```python
from build123d import *

# Parameters (mm, degrees)
SKETCH1_R           = 2
SKETCH1_R_2         = 15
BOSS_EXTRUDE1_DEPTH = 5
FILLET1_R           = 3


with BuildPart() as part:
    # Sketch1 → Boss-Extrude1 (new body)
    with BuildSketch(Plane.XY):
        Polygon((-19.5, -21), (19.5, -21), (19.5, -54), (29.5, -54), (29.5, -17.031832941), (61.515371804, 1.452250588), (56.515371804, 10.112504626), (27.936533479, -6.387495374), (8.436533479, 27.387495374), (37.015371804, 43.887495374), (32.015371804, 52.547749412), (0, 34.063665882), (-32.015371804, 52.547749412), (-37.015371804, 43.887495374), (-8.436533479, 27.387495374), (-27.936533479, -6.387495374), (-56.515371804, 10.112504626), (-61.515371804, 1.452250588), (-29.5, -17.031832941), (-29.5, -54), (-19.5, -54), align=None)
        with Locations((24.5, -24)):
            Circle(SKETCH1_R, mode=Mode.SUBTRACT)
        with Locations((24.5, -29)):
            Circle(SKETCH1_R, mode=Mode.SUBTRACT)
        with Locations((24.5, -34)):
            Circle(SKETCH1_R, mode=Mode.SUBTRACT)
        with Locations((24.5, -39)):
            Circle(SKETCH1_R, mode=Mode.SUBTRACT)
        with Locations((24.5, -44)):
            Circle(SKETCH1_R, mode=Mode.SUBTRACT)
        with Locations((24.5, -49)):
            Circle(SKETCH1_R, mode=Mode.SUBTRACT)
        with Locations(Location((-24.5, -49, 0), (0, 0, 180))):
            Circle(SKETCH1_R, mode=Mode.SUBTRACT)
        with Locations(Location((-24.5, -44, 0), (0, 0, 180))):
            Circle(SKETCH1_R, mode=Mode.SUBTRACT)
        with Locations(Location((-24.5, -39, 0), (0, 0, 180))):
            Circle(SKETCH1_R, mode=Mode.SUBTRACT)
        with Locations(Location((-24.5, -34, 0), (0, 0, 180))):
            Circle(SKETCH1_R, mode=Mode.SUBTRACT)
        with Locations(Location((-24.5, -29, 0), (0, 0, 180))):
            Circle(SKETCH1_R, mode=Mode.SUBTRACT)
        with Locations(Location((-24.5, -24, 0), (0, 0, 180))):
            Circle(SKETCH1_R, mode=Mode.SUBTRACT)
        with Locations(Location((-8.534609691, 33.217622393, 0), (0, 0, 180))):
            Circle(SKETCH1_R, mode=Mode.SUBTRACT)
        with Locations(Location((-12.86473671, 35.717622393, 0), (0, 0, 180))):
            Circle(SKETCH1_R, mode=Mode.SUBTRACT)
        with Locations(Location((-17.194863729, 38.217622393, 0), (0, 0, 180))):
            Circle(SKETCH1_R, mode=Mode.SUBTRACT)
        with Locations(Location((-21.524990748, 40.717622393, 0), (0, 0, 180))):
            Circle(SKETCH1_R, mode=Mode.SUBTRACT)
        with Locations(Location((-25.855117767, 43.217622393, 0), (0, 0, 180))):
            Circle(SKETCH1_R, mode=Mode.SUBTRACT)
        with Locations(Location((-30.185244785, 45.717622393, 0), (0, 0, 180))):
            Circle(SKETCH1_R, mode=Mode.SUBTRACT)
        with Locations((-33.034609691, -9.217622393)):
            Circle(SKETCH1_R, mode=Mode.SUBTRACT)
        with Locations((-37.36473671, -6.717622393)):
            Circle(SKETCH1_R, mode=Mode.SUBTRACT)
        with Locations((-41.694863729, -4.217622393)):
            Circle(SKETCH1_R, mode=Mode.SUBTRACT)
        with Locations((-46.024990748, -1.717622393)):
            Circle(SKETCH1_R, mode=Mode.SUBTRACT)
        with Locations((-50.355117767, 0.782377607)):
            Circle(SKETCH1_R, mode=Mode.SUBTRACT)
        with Locations((-54.685244785, 3.282377607)):
            Circle(SKETCH1_R, mode=Mode.SUBTRACT)
        with Locations(Location((33.034609691, -9.217622393, 0), (0, 0, 180))):
            Circle(SKETCH1_R, mode=Mode.SUBTRACT)
        with Locations(Location((37.36473671, -6.717622393, 0), (0, 0, 180))):
            Circle(SKETCH1_R, mode=Mode.SUBTRACT)
        with Locations(Location((41.694863729, -4.217622393, 0), (0, 0, 180))):
            Circle(SKETCH1_R, mode=Mode.SUBTRACT)
        with Locations(Location((46.024990748, -1.717622393, 0), (0, 0, 180))):
            Circle(SKETCH1_R, mode=Mode.SUBTRACT)
        with Locations(Location((50.355117767, 0.782377607, 0), (0, 0, 180))):
            Circle(SKETCH1_R, mode=Mode.SUBTRACT)
        with Locations(Location((54.685244785, 3.282377607, 0), (0, 0, 180))):
            Circle(SKETCH1_R, mode=Mode.SUBTRACT)
        with Locations((8.534609691, 33.217622393)):
            Circle(SKETCH1_R, mode=Mode.SUBTRACT)
        with Locations((12.86473671, 35.717622393)):
            Circle(SKETCH1_R, mode=Mode.SUBTRACT)
        with Locations((17.194863729, 38.217622393)):
            Circle(SKETCH1_R, mode=Mode.SUBTRACT)
        with Locations((21.524990748, 40.717622393)):
            Circle(SKETCH1_R, mode=Mode.SUBTRACT)
        with Locations((25.855117767, 43.217622393)):
            Circle(SKETCH1_R, mode=Mode.SUBTRACT)
        with Locations((30.185244785, 45.717622393)):
            Circle(SKETCH1_R, mode=Mode.SUBTRACT)
        with Locations((0, 20)):
            Circle(SKETCH1_R, mode=Mode.SUBTRACT)
        with Locations((17.320508076, -10)):
            Circle(SKETCH1_R, mode=Mode.SUBTRACT)
        with Locations((-17.320508076, -10)):
            Circle(SKETCH1_R, mode=Mode.SUBTRACT)
        Circle(SKETCH1_R_2, mode=Mode.SUBTRACT)
    extrude(amount=BOSS_EXTRUDE1_DEPTH)

    # Fillet1
    fillet1_edges = [part.edges().sort_by_distance(p)[0] for p in [
        (19.5, -54, 2.5),
        (19.5, -21, 2.5),
        (-19.5, -21, 2.5),
        (-19.5, -54, 2.5),
        (-29.5, -54, 2.5),
        (-29.5, -17.031832941, 2.5),
        (-61.515371804, 1.452250588, 2.5),
        (-56.515371804, 10.112504626, 2.5),
        (-27.936533479, -6.387495374, 2.5),
        (-8.436533479, 27.387495374, 2.5),
        (-37.015371804, 43.887495374, 2.5),
        (-32.015371804, 52.547749412, 2.5),
        (0, 34.063665882, 2.5),
        (32.015371804, 52.547749412, 2.5),
        (37.015371804, 43.887495374, 2.5),
        (8.436533479, 27.387495374, 2.5),
        (27.936533479, -6.387495374, 2.5),
        (56.515371804, 10.112504626, 2.5),
        (61.515371804, 1.452250588, 2.5),
        (29.5, -17.031832941, 2.5),
        (29.5, -54, 2.5),
    ]]
    fillet(fillet1_edges, radius=FILLET1_R)


solid = part.part
```
Design review of the part built by this model. Coordinates are the model's own, in mm. A direction names the side the tool comes from. Round coordinates to 2 decimals unless told otherwise and drop trailing zeros. Write each loop counter-clockwise with the first axis right and the second up, starting at its lowest first coordinate (ties: lowest second). Pieces come first, ordered by that corner, then holes.
Item 1: The part is to be moulded in two halves that separate along X. For faces 4 (the flat face through (22.56, 35.54, 2.46)), 5 (the cylindrical face through (-15.721, 36.866, 2.465)), say which applies: +X half, -X half, draft (parallel to the pull), parting line (faces both ways), or undercut.
Item 2: Clearance check with a flat-ended pin moving along its axis: pin 1 Ø2 at (y, z) = (-25, 2.5) entering from +X. State where the tip first meets the part, or that it passes through.
Item 3: We need section C-C on y = 20. Write out the cut boundary in (x, z), and give its area (3 significant figures).
Item 4: We need section A-A on x = 0. Write out the cut boundary in (y, z).
Item 5: We need section B-B on y = -29. Write out the cut boundary in (x, z).
Item 6: For probe 1 along Y at (x, z) = (-21, 2.2); probe 2 along Y at (x, z) = (-16, 2.95); probe 3 along X at (y, z) = (47, 2.7), list the stretches that pass through material, from the lowest coordinate up.
Item 7: For faces 1 (the cylindrical face through (18.6, -21.86, 2.54)), 2 (the flat face through (18.3, 10.3, 2.5)), 3 (the flat face through (44.8, -8.2, 2.5)), list the 3-axis set-ups (+Z, -Z, +X, -X, +Y, -Y) from which the entire face can be reached by the end or side of a thin tool; tool diameter is ignored.
Item 8: We need section D-D on x = 42. Write out the cut boundary in (y, z), and give its area (3 significant figures).
Returned:
1. face 4: +X half
1. face 5: undercut
2. pin 1: stops at x = 29.5
3. outline: (-12.7, 0) - (-2, 0) - (-2, 5) - (-12.7, 5) - close; (2, 0) - (12.7, 0) - (12.7, 5) - (2, 5) - close
3. area: 107 mm2
4. outline: (-21, 0) - (-15, 0) - (-15, 5) - (-21, 5) - close; (15, 0) - (18, 0) - (18, 5) - (15, 5) - close; (22, 0) - (34.53, 0) - (34.53, 5) - (22, 5) - close
5. outline: (-29.5, 0) - (-26.5, 0) - (-26.5, 5) - (-29.5, 5) - close; (-22.5, 0) - (-19.5, 0) - (-19.5, 5) - (-22.5, 5) - close; (19.5, 0) - (22.5, 0) - (22.5, 5) - (19.5, 5) - close; (26.5, 0) - (29.5, 0) - (29.5, 5) - (26.5, 5) - close
6. probe 1: y = -53.6 to 5.63, 34.64 to 38.79, 42.65 to 46.19
6. probe 2: y = -21 to -11.5, -8.5 to 14.29, 31.75 to 36.61, 39.82 to 43.3
6. probe 3: x = -35.22 to -31.72, -28.65 to -22.41, 22.41 to 28.65, 31.72 to 35.22
7. face 1: +Z, -Z, -Y
7. face 2: +Z, -Z
7. face 3: +Z, -Z, +X, -Y
8. outline: (-9.81, 0) - (-6.19, 0) - (-6.19, 5) - (-9.81, 5) - close; (-2.24, 0) - (1.73, 0) - (1.73, 5) - (-2.24, 5) - close
8. area: 38.0 mm2
